Autodesk Inventor part; units mm, degrees
ref_plane "IDS_WORKPLANE{1}" through (-2.1389, 0, 0) normal (1, 0, 0) x (0, 0, -1)
ref_plane "Work Plane2" through (8.25, 0, 0) normal (0, 0, -1) x (1, 0, 0)
ref_plane "YZ Plane" through (0, 0, 0) normal (1, 0, 0) x (0, 1, 0)
sketch "Skizze1" plane through (0, 0, 0) normal (0, 0, 1) x (1, 0, 0)
  line L0 (-2.1389, 0) -> (5, 0)
  line L1 (5, 0) -> (5, 1.5)
  line L2 (5, 1.5) -> (1.25, 1.5)
  line L3 (1.25, 1.5) -> (0.9433, 1.3468)
  line L4 (0.9433, 1.3468) -> (0, 1.3467)
  line L5 (0, 1.3467) -> (0, 2.75)
  line L6 (-6.0203, 0) -> (20.8022, 0)
  line L7 (0, -0.5507) -> (0, 3.3039)
  line L8 (0, 2.75) -> (-1.94, 2.7497)
  arc A0 (-1.94, 2.7497) -> (-2.1389, 0) centre (16.9704, 0) ccw
  dimension "d0" = 5
  dimension "d1" = 3.75
  dimension "d2" = 0.3067
  dimension "d3" = 2.1389
  dimension "d4" = 3
  dimension "d5" = 2.6935
  dimension "d9" = 5.5
  dimension "d10" = 0.01
  dimension "d15" = 19.1093
revolve "Körper" add sketch "Skizze1" angle 360 about axis through (-2.1389, 0, 0) along (1, 0, 0)
fillet "Rundung1" radius 1.8 1 edges at (-1.94, -2.7497, 0)
ref_plane "IDS_WORKPLANE{1}" through (-2.1389, 0, 0) normal (1, 0, 0) x (0, 0, -1)
sketch "Skizze2" plane through (-2.1389, 0, 0) normal (1, 0, 0) x (0, 0, -1)
  line L0 (0, -3.85) -> (0, 3.85)
  line L1 (3.85, 0) -> (-3.85, 0)
  line L2 (-2.75, 0.4) -> (2.75, 0.4)
  line L3 (2.75, 0.4) -> (2.75, -0.4)
  line L4 (2.75, -0.4) -> (-2.75, -0.4)
  line L5 (-2.75, -0.4) -> (-2.75, 0.4)
  line L6 (0, 0.4) -> (0, -0.4) construction
  line L7 (-2.75, 0) -> (2.75, 0) construction
  circle A0 centre (0, 0) radius 2.75
  dimension "d17" = 0.8
extrude "Loch" cut sketch "Skizze2" along normal blind 1.2 contours L4 A0 L1 L0 | L0 L1 A0 L4 | L4 L5 A0 | A0 L3 L4 | L1 A0 L2 L0 | L0 L2 A0 L1 | L5 L2 A0 | A0 L2 L3
thread "Gewinde"
chamfer "Fase1" distance 0.3067 distance2 0.3068 1 edges at (5, -1.5, 0) measured on face at (5, 0.8773, -0.3972)
ref_plane "Work Plane2" through (8.25, 0, 0) normal (0, 0, -1) x (1, 0, 0)
equation "\"d0\" = NLG"
equation "\"d1\" = GEL"
equation "\"d2\" = GAL"
equation "\"d3\" = KOH"
equation "\"d4\" = GD"
equation "\"d5\" = BDM"
equation "\"d9\" = KOD"
equation "\"d10\" = KEWI"
equation "\"d17\" = SBR"
equation "\"d18\" = STI"
equation "\"d20\" = RR"
equation "\"d11\" = GEL"
equation "\"d13\" = -0.5 * SPD + 0.5 * GD"
equation "\"GD\" = NND"
equation "\"NLG\" = 5"
equation "\"GEL\" = 3.75"
equation "\"KOD\" = 5.5"
equation "\"KOH\" = 2.13889"
equation "\"GAL\" = 0.61345 * PTC"
equation "\"SPD\" = NND - 1.2269 * PTC"
equation "\"BDM\" = 2.6935"
equation "\"GUL\" = 0.61345 * PTC"
equation "\"RR\" = 1.8"
equation "\"SBR\" = 0.8"
equation "\"STI\" = 1.2"
equation "\"KEWI\" = 0.01deg"
equation "\"KR\" = 3.3"
equation "\"d16\" = -KOH"
equation "\"PTC\" = 0.5"
equation "\"THREADDIA\" = 3"
equation "\"TOA\" = 30deg"
equation "\"NND\" = 3"
equation "\"ORI\" = 1.8"
equation "\"GD1\" = THREADDIA - 1.2269 * PTC"
properties part number "CNS 9671 - M3 x 5" material "Steel, Mild"
Input: part model. Units: mm. Frame: model coordinates. A direction names the side the tool comes from. Coordinates: 2 decimals unless noted, no trailing zeros. Loops run counter-clockwise (first coordinate to the right, second up) from the corner with the lowest first, then second, coordinate; pieces in that order, holes last. Notation, with made-up numbers: M 86,36 L 135,36 A25 ccw 135,59 Z; hole C 20,3 d7. An arc over 180 degrees is marked long. Use a Markdown table: item, result. Add a question column.
1) Set-up query: faces 5 (the cylindrical face through (0.465, 1.244, 0.516)), 6 (the flat face through (-1.5, 0.4, 0)), 7 (the cylindrical face through (-0.159, -0.596, 2.685)). Return all of +Z, -Z, +X, -X, +Y, -Y with unobstructed straight access to the full face (end or side cutting, diameter ignored); none if empty.
2) Section A-A, the plane x = 3.75. Return the cut outline in (y, z).
3) Pin query (flat end, axial travel): P1, Ø3, axis at x = -0.5, y = 2, coming from the +Z side; P2, Ø1.3, axis at x = -1.5, z = 0, coming from the +Y side; P3, Ø1.3, axis at x = -1.5, z = 0.5, coming from the -Y side. Return the tip coordinate at first contact, or that it passes through.
4) Line query: L1, parallel to Y at x = -0.5, z = 0.75; L2, parallel to Y at x = -1.5, z = -1.55; L3, parallel to X at y = 0.15, z = 0.05. Output: solid intervals per line, ascending. Write a range as from..to.
5) Draft query along Y for faces 1 (the flat face through (-1.5, -0.4, 0)), 2 (the flat face through (5, 0, 0)), 3 (the flat face through (-0.939, 0, 0)), 4 (the cylindrical face through (2.95, -1.5, -0.07)). Return one class per face: +Y half, -Y half, draft (parallel to the pull), parting line (faces both ways), or undercut.
Answer below:
| question | item | result |
|---|---|---|
| 1 | face 5 | none |
| 1 | face 6 | +Z, -Z, -X |
| 1 | face 7 | +X, -X |
| 2 | outline | C 0,0 d3 |
| 3 | P1 | z = 2.7 |
| 3 | P2 | y = 2.67 |
| 3 | P3 | y = -2.64 |
| 4 | L1 | -2.64..2.64 |
| 4 | L2 | -1.7..-0.4, 0.4..1.7 |
| 4 | L3 | -0.94..5 |
| 5 | face 1 | undercut |
| 5 | face 2 | draft |
| 5 | face 3 | undercut |
| 5 | face 4 | parting line |
